The listing builds one solid part. Answer for the finished solid, in the listing's coordinates (mm). Face numbers are marked on the shaded views. A direction names the side the tool comes from. Coordinates: 2 decimals unless noted, no trailing zeros. Write each loop counter-clockwise with the first axis right and the second up, starting at its lowest first coordinate (ties: lowest second). Pieces come first, ordered by that corner, then holes. Notation, with made-up numbers: M 21,87.25 L 68,87.25 A30 ccw 68,119.25 Z; hole C -35,-5.5 d6. An arc over 180 degrees is marked long. Answer as a JSON object with one key per item and string values. Group by question number.
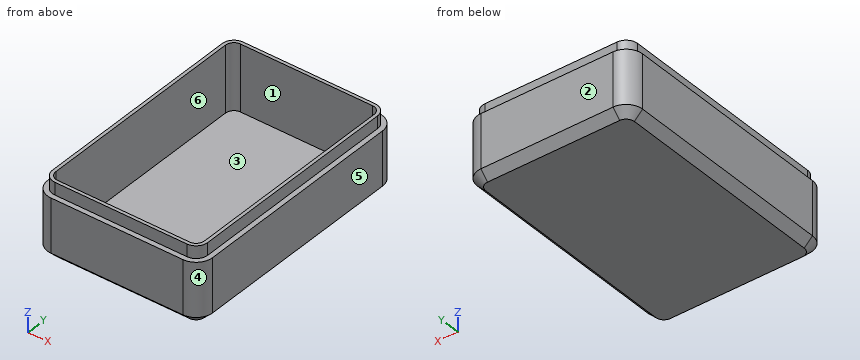
from build123d import *

# Parameters (mm, degrees)
PAD_DEPTH    = 15
POCKET_DEPTH = 13
PAD001_DEPTH = 3
CHAMFER_SIZE = 2


with BuildPart() as part:
    # Sketch → Pad (new body)
    with BuildSketch(Plane.XY):
        with BuildLine():
            Line((-20, 26), (-20, -26))
            ThreePointArc((-20, -26), (-18.828427, -28.828427), (-16, -30))
            Line((-16, -30), (16, -30))
            ThreePointArc((16, -30), (18.828427, -28.828427), (20, -26))
            Line((20, -26), (20, 26))
            ThreePointArc((20, 26), (18.828427, 28.828427), (16, 30))
            Line((16, 30), (-16, 30))
            ThreePointArc((-16, 30), (-18.828427, 28.828427), (-20, 26))
        make_face()
    extrude(amount=PAD_DEPTH)

    # Sketch001 (on Face10 of Pad) → Pocket (cut)
    with BuildSketch(Plane.XY.offset(15)):
        with BuildLine():
            Line((-18, 26), (-18, -26))
            ThreePointArc((-18, -26), (-17.414214, -27.414214), (-16, -28))
            Line((-16, -28), (16, -28))
            ThreePointArc((16, -28), (17.414214, -27.414214), (18, -26))
            Line((18, -26), (18, 26))
            ThreePointArc((18, 26), (17.414214, 27.414214), (16, 28))
            Line((16, 28), (-16, 28))
            ThreePointArc((-16, 28), (-17.414214, 27.414214), (-18, 26))
        make_face()
    extrude(amount=-POCKET_DEPTH, mode=Mode.SUBTRACT)

    # Sketch002 (on Face5 of Pocket) → Pad001 (join)
    with BuildSketch(Plane.XY.offset(15)):
        with BuildLine():
            Line((-18.8, 26), (-18.8, -26))
            ThreePointArc((-18.8, -26), (-17.979899, -27.979899), (-16, -28.8))
            Line((-16, -28.8), (16, -28.8))
            ThreePointArc((16, -28.8), (17.979899, -27.979899), (18.8, -26))
            Line((18.8, -26), (18.8, 26))
            ThreePointArc((18.8, 26), (17.979899, 27.979899), (16, 28.8))
            Line((16, 28.8), (-16, 28.8))
            ThreePointArc((-16, 28.8), (-17.979899, 27.979899), (-18.8, 26))
        make_face()
        with BuildLine():
            Line((-18, 26), (-18, -26))
            ThreePointArc((-18, -26), (-17.414214, -27.414214), (-16, -28))
            Line((-16, -28), (16, -28))
            ThreePointArc((16, -28), (17.414214, -27.414214), (18, -26))
            Line((18, -26), (18, 26))
            ThreePointArc((18, 26), (17.414214, 27.414214), (16, 28))
            Line((16, 28), (-16, 28))
            ThreePointArc((-16, 28), (-17.414214, 27.414214), (-18, 26))
        make_face(mode=Mode.SUBTRACT)
    extrude(amount=PAD001_DEPTH)

    # Chamfer
    chamfer_edges = [part.edges().sort_by_distance(p)[0] for p in [
        (0, -30, 0),
        (18.828427, -28.828427, 0),
        (20, 0, 0),
        (18.828427, 28.828427, 0),
        (0, 30, 0),
        (-18.828427, 28.828427, 0),
        (-20, 0, 0),
        (-18.828427, -28.828427, 0),
    ]]
    chamfer(chamfer_edges, length=CHAMFER_SIZE)


solid = part.part
Item 1: A cutting plane is placed at A-A, the plane z = 12. Write down the section's boundary in (x, y), and give its area (3 significant figures).
Item 2: A cutting plane is placed at C-C, the plane y = -20. Write down the section's boundary in (x, z), and give its area (3 significant figures).
Item 3: A cutting plane is placed at D-D, the plane z = 15.75. Write down the section's boundary in (x, y), and give its area (3 significant figures).
Item 4: Flat-ended cylindrical pins translate along their axes: pin 1 Ø2.5 at (y, z) = (-1.5, 16.5) entering from +X; pin 2 Ø1.5 at (x, z) = (-8, 17) entering from +Y; pin 3 Ø1.5 at (x, z) = (1.5, 17) entering from -Y. Find the tip coordinate at first contact, or state that the pin passes through.
Item 5: A tool of negligible diameter and unlimited length cuts with its end or side. For the marked faces 5 and 6, from which of +Z, -Z, +X, -X, +Y, -Y can it reach the whole face along a straight path? Write none if from no direction.
Item 6: Consider L1, parallel to Y at x = 7.5, z = 14.5; L2, parallel to X at y = -24, z = 8.5; L3, parallel to Z at x = 7, y = -24. Determine where each line is inside the solid, lowest interval first. Write a range as from..to.
Item 7: A cutting plane is placed at B-B, the plane x = -1.5. Write down the section's boundary in (y, z), and give its area (3 significant figures).
Item 8: For a pull along X with two mould halves and no side action, classify the marked faces 1, 2, 3 and 4 as +X half, -X half, draft (parallel to the pull), parting line (faces both ways), or undercut.
Answer:
{
 "1": {"outline": "M -20,-26 A4 ccw -16,-30 L 16,-30 A4 ccw 20,-26 L 20,26 A4 ccw 16,30 L -16,30 A4 ccw -20,26 Z; hole M -18,-26 A2 ccw -16,-28 L 16,-28 A2 ccw 18,-26 L 18,26 A2 ccw 16,28 L -16,28 A2 ccw -18,26 Z", "area": "374 mm2"},
 "2": {"outline": "M -20,2 L -18,0 L 18,0 L 20,2 L 20,15 L 18.8,15 L 18.8,18 L 18,18 L 18,2 L -18,2 L -18,18 L -18.8,18 L -18.8,15 L -20,15 Z", "area": "133 mm2"},
 "3": {"outline": "M -18.8,-26 A2.8 ccw -16,-28.8 L 16,-28.8 A2.8 ccw 18.8,-26 L 18.8,26 A2.8 ccw 16,28.8 L -16,28.8 A2.8 ccw -18.8,26 Z; hole M -18,-26 A2 ccw -16,-28 L 16,-28 A2 ccw 18,-26 L 18,26 A2 ccw 16,28 L -16,28 A2 ccw -18,26 Z", "area": "146 mm2"},
 "4": {"pin 1": "x = 18.8", "pin 2": "y = 28.8", "pin 3": "y = -28.8"},
 "5": {"face 5": "+Z, -Z, +X, +Y, -Y", "face 6": "+Z"},
 "6": {"L1": "-30..-28, 28..30", "L2": "-20..-18, 18..20", "L3": "0..2"},
 "7": {"outline": "M -30,2 L -28,0 L 28,0 L 30,2 L 30,15 L 28.8,15 L 28.8,18 L 28,18 L 28,2 L -28,2 L -28,18 L -28.8,18 L -28.8,15 L -30,15 Z", "area": "173 mm2"},
 "8": {"face 1": "undercut", "face 2": "draft", "face 3": "undercut", "face 4": "+X half"}
}
